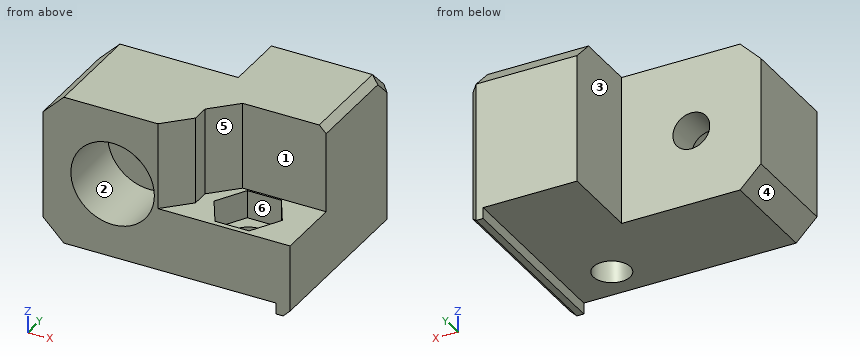
from build123d import *

# Parameters (mm, degrees)
SKETCH_W        = 13.5
SKETCH_H        = 26.5
SKETCH_R        = 2.65
PAD_DEPTH       = 5
PAD001_DEPTH    = 4
SKETCH002_W     = 13.5
SKETCH002_H     = 17
PAD002_DEPTH    = 16.5
SKETCH003_W     = 20
SKETCH003_H     = 21.5
SKETCH003_R     = 2.65
PAD003_DEPTH    = 14.75
SKETCH004_R     = 6
POCKET_DEPTH    = 9.75
PAD004_DEPTH    = 2
CHAMFER_SIZE    = 3
CHAMFER001_SIZE = 3.5
CHAMFER002_SIZE = 1


with BuildPart() as part:
    # Sketch → Pad (new body)
    with BuildSketch(Plane.XY):
        with Locations((6.75, 13.25)):
            Rectangle(SKETCH_W, SKETCH_H)
        with Locations((6.75, 5)):
            Circle(SKETCH_R, mode=Mode.SUBTRACT)
    extrude(amount=-PAD_DEPTH)

    # Sketch001 → Pad001 (join)
    with BuildSketch(Plane.XY):
        Polygon((0, 0), (4.729274, 0), (8.770726, 0), (13.5, 0), (13.5, 26.5), (0, 26.5), align=None)
        Polygon((9.203739, 0.75), (11.657477, 5), (9.203739, 9.25), (4.296261, 9.25), (1.842523, 5), (4.296261, 0.75), align=None, mode=Mode.SUBTRACT)
    extrude(amount=PAD001_DEPTH)

    # Sketch002 → Pad002 (join)
    with BuildSketch(Plane.XY):
        with Locations((6.75, 18)):
            Rectangle(SKETCH002_W, SKETCH002_H)
    extrude(amount=PAD002_DEPTH)

    # Sketch003 (on DatumPlane) → Pad003 (join)
    with BuildSketch(Plane.XZ.offset(-14.75)):
        with Locations((-10, 5.75)):
            Rectangle(SKETCH003_W, SKETCH003_H)
        with Locations((-10, 5.75)):
            Circle(SKETCH003_R, mode=Mode.SUBTRACT)
    extrude(amount=PAD003_DEPTH)

    # Sketch004 → Pocket (cut)
    with BuildSketch(Plane.XZ):
        with Locations((-10, 5.75)):
            Circle(SKETCH004_R)
    extrude(amount=-POCKET_DEPTH, mode=Mode.SUBTRACT)

    # Sketch005 (on DatumPlane) → Pad004 (join)
    with BuildSketch(Plane.YZ.offset(13.5)):
        Polygon((0, 0), (0, -6.6), (26.5, -6.6), (26.5, 16.5), (9.5, 16.5), (9.5, 4), (0, 4), align=None)
    extrude(amount=PAD004_DEPTH)

    # Chamfer
    chamfer_edges = [part.edges().sort_by_distance(p)[0] for p in [
        (6.75, 26.5, 16.5),
        (14.5, 26.5, 16.5),
        (-20, 7.375, -5),
        (-20, 7.375, 16.5),
    ]]
    chamfer(chamfer_edges, length=CHAMFER_SIZE)

    # Chamfer001
    chamfer001_edges = [part.edges().sort_by_distance(p)[0] for p in [
        (0, 9.5, 10.25),
        (0, 0, 10.25),
    ]]
    chamfer(chamfer001_edges, length=CHAMFER001_SIZE)

    # Chamfer002
    chamfer002_edges = [part.edges().sort_by_distance(p)[0] for p in [
        (15.5, 16.5, 16.5),
        (15.5, 13.25, -6.6),
        (15.5, 25, 15),
        (15.5, 26.5, 3.45),
    ]]
    chamfer(chamfer002_edges, length=CHAMFER002_SIZE)


solid = part.part
Geometry: final body of the model. Coordinates: model frame, mm. Face numbers are marked on the shaded views. A direction names the side the tool comes from. Round coordinates to 2 decimals unless told otherwise and drop trailing zeros. Loops run counter-clockwise (first coordinate to the right, second up) from the corner with the lowest first, then second, coordinate; pieces in that order, holes last.
Q1. Pull-direction query (Y, two-part tool) for the marked faces 4, 5 and 6; classes: released by +Y, released by -Y, zero draft, split by the parting line, or undercut.
Q2. Pin query (flat end, axial travel): P1, Ø4, axis at x = 8, y = 3.5, coming from the +Z side; P2, Ø6, axis at x = -12.5, z = 5.5, coming from the -Y side; P3, Ø3, axis at y = 21.5, z = -1.5, coming from the -X side. Return the tip coordinate at first contact, or that it passes through.
Q3. Section A-A on z = 5.75. Return loops of the section in (x, y), plus the area to 4 significant figures.
Q4. Access query for the marked faces 1, 2 and 3. Directions: +Z, -Z, +X, -X, +Y, -Y. A direction counts if a zero-diameter tool reaches every point of the face in a straight line with its end or side. Return the directions, or none.
Q5. Section B-B on x = -10. Return loops of the section in (y, z), plus the area to 3 significant figures.
Q6. Section D-D on x = 13. Return loops of the section in (y, z), plus the area to 4 significant figures.
Q7. Material intervals for L1, parallel to X at y = 2.75, z = 2; L2, parallel to Y at x = 6.75, z = -1.5; L3, parallel to X at y = 2.25, z = 3, sorted ascending.
Q8. Section C-C on y = 10.25. Return loops of the section in (x, z).
Evaluation:
1. face 4: zero draft
1. face 5: released by -Y
1. face 6: undercut
2. P1: stops at z = 0
2. P2: stops at y = 9.75
2. P3: stops at x = 0
3. outline: (-20, 0) - (-16, 0) - (-16, 9.75) - (-12.65, 9.75) - (-12.65, 14.75) - (-20, 14.75) - close; (-7.35, 9.75) - (-4, 9.75) - (-4, 0) - (-3.5, 0) - (0, 3.5) - (0, 6) - (3.5, 9.5) - (15.5, 9.5) - (15.5, 25.5) - (14.5, 26.5) - (0, 26.5) - (0, 14.75) - (-7.35, 14.75) - close
3. area: 414.5 mm2
4. face 1: +Z, +X, -Y
4. face 2: -Y
4. face 3: +Z, -Z, -X, +Y
5. outline: (0, -5) - (14.75, -5) - (14.75, 3.1) - (9.75, 3.1) - (9.75, -0.25) - (0, -0.25) - close; (0, 11.75) - (9.75, 11.75) - (9.75, 8.4) - (14.75, 8.4) - (14.75, 16.5) - (0, 16.5) - close
5. area: 174 mm2
6. outline: (0, -5) - (26.5, -5) - (26.5, 13.5) - (23.5, 16.5) - (9.5, 16.5) - (9.5, 4) - (0, 4) - close
6. area: 446.5 mm2
7. L1: x = -20 to -14.68, -5.32 to 3.14, 10.36 to 15.5
7. L2: y = 0 to 2.35, 7.65 to 26.5
7. L3: x = -20 to -15.33, -4.67 to 3.43, 10.07 to 15.5
8. outline: (-20, -2) - (-17, -5) - (13.5, -5) - (13.5, -6.6) - (14.5, -6.6) - (15.5, -5.6) - (15.5, 15.5) - (14.5, 16.5) - (-17, 16.5) - (-20, 13.5) - close; hole circle Ø5.3 at (-10, 5.75)
